from build123d import *

# Parameters (mm, degrees)
F1_W     = 19
F1_H     = 19
F1_W_2   = 16.6
F1_H_2   = 16.6
F2_DEPTH = 500
F4_D     = 5
F6_D     = 5


with BuildPart() as f2:
    # F1 (on Front) → F2 (new body)
    with BuildSketch(Plane.XZ):
        Rectangle(F1_W, F1_H)
        Rectangle(F1_W_2, F1_H_2, mode=Mode.SUBTRACT)
    extrude(amount=-F2_DEPTH)

    # F4 (through all)
    with Locations(Plane.XY.offset(9.5)):
        with Locations((0, 490), (0, 470)):
            Hole(F4_D / 2)

    # F6 (through all)
    with Locations(Plane.YZ.offset(9.5)):
        with Locations((10, 0), (60, 0)):
            Hole(F6_D / 2)


solid = f2.part
The listing builds one solid part. Answer for the finished solid, in the listing's coordinates (mm). A direction names the side the tool comes from. Give positions to 0.01 mm unless a question says otherwise; leave off trailing zeros. Write each loop counter-clockwise with the first axis right and the second up, starting at its lowest first coordinate (ties: lowest second). Pieces come first, ordered by that corner, then holes.
1) For a pull along Z with two mould halves and no side action, classify faces 1 (the face through (0, 246, 9.5)), 2 (the face through (0, 246, -9.5)), 3 (the face through (9.5, 246, 0)), 4 (the face through (0, 246, 8.3)) as pulls with the +Z half, pulls with the -Z half, needs draft (parallel to the pull), parting line crosses it, or undercut.
2) Find the intervals of material crossed by L1, parallel to X at y = 90, z = 1.75; L2, parallel to Y at x = 0, z = -8.9, in increasing order.
3) A tool of negligible diameter and unlimited length cuts with its end or side. For faces 5 (the face through (-9, 0, 0)), 6 (the face through (0, 246, -8.3)), from which of +Z, -Z, +X, -X, +Y, -Y can it reach the whole face along a straight path? Write none if from no direction.
4) Section A-A (y = 145) is taken. Write down the section's boundary in (x, z).
5) Given P1, Ø3, axis at x = 0, y = 470, coming from the -Z side, flat-ended and moving along its own axis, determine where the tip first touches the part or whether it passes through.
Response:
1. face 1: pulls with the +Z half
1. face 2: pulls with the -Z half
1. face 3: needs draft
1. face 4: undercut
2. L1: x = -9.5 to -8.3, 8.3 to 9.5
2. L2: y = 0 to 467.5, 472.5 to 487.5, 492.5 to 500
3. face 5: +Z, -Z, +X, -X, -Y
3. face 6: +Y, -Y
4. outline: (-9.5, -9.5) - (9.5, -9.5) - (9.5, 9.5) - (-9.5, 9.5) - close; hole (-8.3, -8.3) - (8.3, -8.3) - (8.3, 8.3) - (-8.3, 8.3) - close
5. P1: passes through
